Can you work these out from the drawing? Everything is in mm from the part's minimum corner. A direction names the side the tool comes from. Give positions to 0.01 mm unless a question says otherwise; leave off trailing zeros. Order: outer loops, then holes, each group sorted by start corner. A loop starts at its lowest first (then second) coordinate and runs counter-clockwise, first axis right, second up. Notation, with made-up numbers: M 87,81.25 L 123,81.25 A8 cw 123,94.25 Z; hole C -35,-27 d2. An arc over 180 degrees is marked long. Answer in a Markdown table with one row per item. Add a question column.
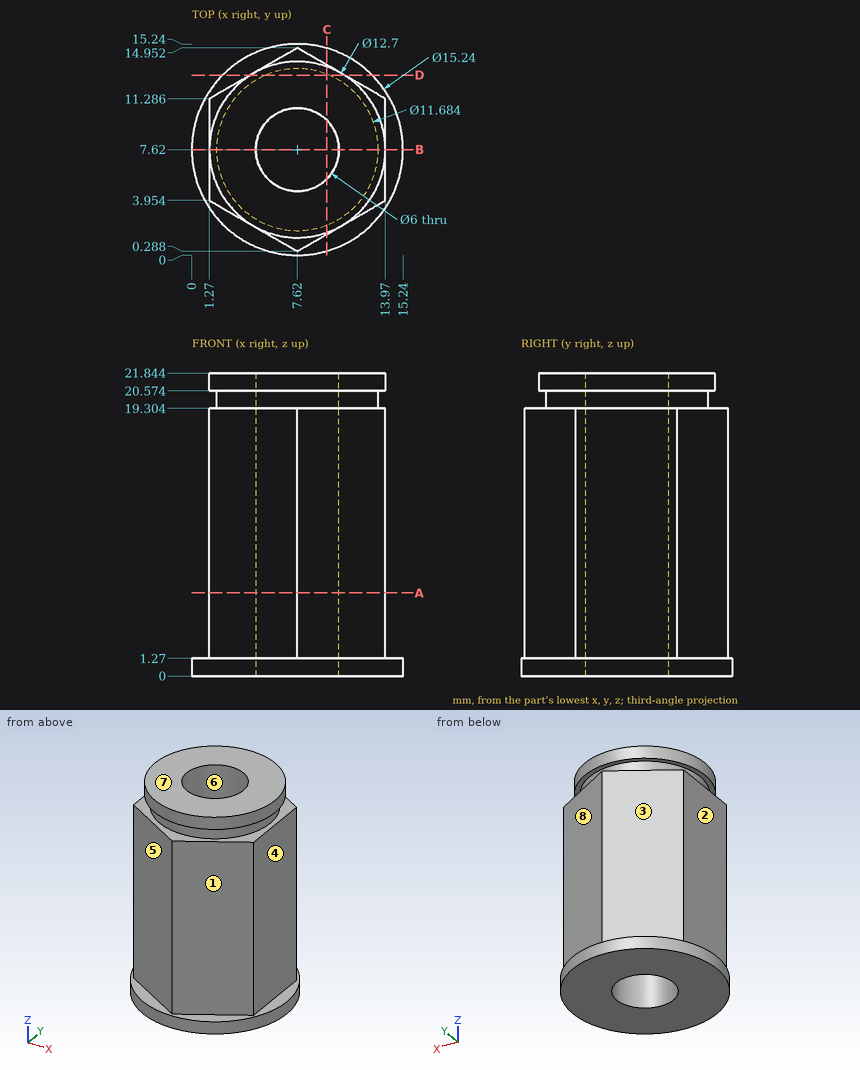
1. Suppose I cut it at A-A on z = 6. List the corners of the cut face in (x, y) for me.
2. For the marked faces 1, 2, 3, 4 and 5, which set-ups out of +Z, -Z, +X, -X, +Y, -Y let a thin tool reach every point of the face, with its end or its side?
3. Will these pins go through, and if not, where does the flat tip stop? P1, Ø8, axis at y = 7.5, z = 14.5, coming from the +X side; P2, Ø2, axis at x = 13.5, z = 2.5, coming from the +Y side (1 decimal); P3, Ø6, axis at y = 7.5, z = 7.5, coming from the -X side; P4, Ø6, axis at y = 8.5, z = 3.5, coming from the +X side.
4. Suppose I cut it at B-B on y = 7.62. List the corners of the cut face in (x, z) for me, plus the area to 3 significant figures.
5. Suppose I cut it at C-C on x = 9.75. List the corners of the cut face in (y, z) for me.
6. Thinking about a two-plate mould opening in Y: for the marked faces 6, 7 and 8, which applies, pulls with the +Y half, pulls with the -Y half, needs draft (parallel to the pull), parting line crosses it, or undercut?
7. If I drill on line 1 along Z through (x, y) = (11.25, 3); line 2 along X through (y, z) = (7.62, 14.75); line 3 along Z through (x, y) = (4.5, 2), over which ranges is the centre line in solid material (lowest first)? Write a range as [from, to].
8. Suppose I cut it at D-D on y = 13. List the corners of the cut face in (x, z) for me.
Findings below:
| question | item | result |
|---|---|---|
| 1 | outline | M 1.27,3.95 L 7.62,0.29 L 13.97,3.95 L 13.97,11.29 L 7.62,14.95 L 1.27,11.29 Z; hole C 7.62,7.62 d6 |
| 2 | face 1 | +Z, +X, -Y |
| 2 | face 2 | +Z, -X, +Y, -Y |
| 2 | face 3 | +Z, -X, +Y |
| 2 | face 4 | +Z, +X, +Y, -Y |
| 2 | face 5 | +Z, -X, -Y |
| 3 | P1 | x = 13.97 |
| 3 | P2 | y = 12.1 |
| 3 | P3 | x = 1.27 |
| 3 | P4 | x = 15.24 |
| 4 | outline | M 0,0 L 4.62,0 L 4.62,21.84 L 1.27,21.84 L 1.27,20.57 L 1.78,20.57 L 1.78,19.3 L 1.27,19.3 L 1.27,1.27 L 0,1.27 Z; M 10.62,0 L 15.24,0 L 15.24,1.27 L 13.97,1.27 L 13.97,19.3 L 13.46,19.3 L 13.46,20.57 L 13.97,20.57 L 13.97,21.84 L 10.62,21.84 Z |
| 4 | area | 148 mm2 |
| 5 | outline | M 0.3,0 L 5.51,0 L 5.51,21.84 L 1.64,21.84 L 1.64,20.57 L 2.18,20.57 L 2.18,19.3 L 1.52,19.3 L 1.52,1.27 L 0.3,1.27 Z; M 9.73,0 L 14.94,0 L 14.94,1.27 L 13.72,1.27 L 13.72,19.3 L 13.06,19.3 L 13.06,20.57 L 13.6,20.57 L 13.6,21.84 L 9.73,21.84 Z |
| 6 | face 6 | undercut |
| 6 | face 7 | needs draft |
| 6 | face 8 | pulls with the +Y half |
| 7 | line 1 | [0, 19.3], [20.57, 21.84] |
| 7 | line 2 | [1.27, 4.62], [10.62, 13.97] |
| 7 | line 3 | [0, 1.27] |
| 8 | outline | M 2.22,0 L 13.02,0 L 13.02,1.27 L 11,1.27 L 11,19.3 L 9.9,19.3 L 9.9,20.57 L 10.99,20.57 L 10.99,21.84 L 4.25,21.84 L 4.25,20.57 L 5.34,20.57 L 5.34,19.3 L 4.24,19.3 L 4.24,1.27 L 2.22,1.27 Z |
